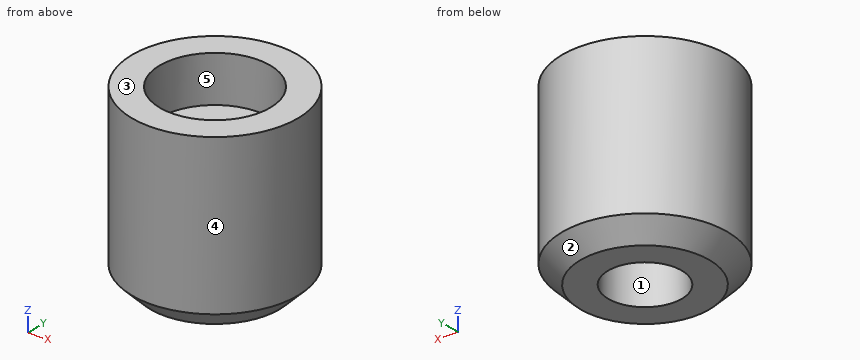
Autodesk Inventor part; units mm, degrees
ref_plane "YZ Plane" through (0, 0, 0) normal (1, 0, 0) x (0, 1, 0)
ref_plane "XZ Plane" through (0, 0, 0) normal (0, 1, 0) x (-1, 0, 0)
ref_plane "XY Plane" through (0, 0, 0) normal (0, 0, 1) x (1, 0, 0)
sketch "Skizze1" plane through (0, 0, 0) normal (0, 0, 1) x (1, 0, 0)
  circle A0 centre (0, 0) radius 2
  circle A1 centre (0, 0) radius 4.5
  dimension "d0" = 9
  dimension "d1" = 4
extrude "Extrusion1" add sketch "Skizze1" along normal blind 9.5
sketch "Skizze2" plane through (0, 0, 9.5) normal (0, 0, 1) x (1, 0, 0)
  circle A0 centre (0, 0) radius 3
  dimension "d4" = 6
extrude "Extrusion2" cut sketch "Skizze2" against normal blind 2.5
chamfer "Fase1" distance 1 angle 45 1 edges at (-4.5, 0, 0)
sketch "Skizze3" plane through (0, 0, 7) normal (0, 0, 1) x (1, 0, 0)
  circle A0 centre (0, 0) radius 2
  circle A1 centre (0, 0) radius 3
extrude "Extrusion3" add sketch "Skizze3" against normal blind 0.4 contours A0
properties part number "Mag4mmWelle" material "ABS-Kunststoff"
Verification items for the finished model (mm, model axes). Face numbers are marked on the shaded views. A direction names the side the tool comes from. Coordinates: 2 decimals unless noted, no trailing zeros. Order: outer loops, then holes, each group sorted by start corner. A loop starts at its lowest first (then second) coordinate and runs counter-clockwise, first axis right, second up. Notation, with made-up numbers: M 65.25,35 L 73.25,35 A35 cw 73.25,71 Z; hole C 75,-2 d7. An arc over 180 degrees is marked long. One line per item, written item: value. Start each with the question number.
Item 1: Sectioned sample at C-C on z = 8.5. Record the cut outline in (x, y), then the cut area to 3 significant figures.
Item 2: Access from +Z, -Z, +X, -X, +Y, -Y to the whole of each face (thin tool, end or side, straight path). Record for the marked faces 4 and 5.
Item 3: Sectioned sample at A-A on x = 0. Record the cut outline in (y, z).
Item 4: Mould release check, pull along Y, two halves, no side actions. Record for the marked faces 1, 2 and 3: pulls with the +Y half, pulls with the -Y half, needs draft (parallel to the pull), parting line crosses it, or undercut.
Item 5: Sectioned sample at B-B on z = 5.25. Record the cut outline in (x, y), then the cut area to 3 significant figures.
Item 6: Depth check by flat-ended pin: P1, Ø1, axis at x = -2, z = 5.5, coming from the -Y side; P2, Ø3.5, axis at x = 0, y = 0, coming from the +Z side; P3, Ø1.2, axis at x = 0.5, y = -0.5, coming from the -Z side. Enter the tip coordinate at first touch or a pass-through.
Item 7: Thickness scan on probe 1 along Y at (x, z) = (0, 7.85); probe 2 along Z at (x, y) = (-1.75, -0.75); probe 3 along Y at (x, z) = (0, 3.75). Record the ranges inside material, lowest first.
Calculated:
1. outline: C 0,0 d9; hole C 0,0 d6
1. area: 35.3 mm^2
2. face 4: +Z, -Z
2. face 5: +Z
3. outline: M -4.5,1 L -3.5,0 L -2,0 L -2,6.6 L 2,6.6 L 2,0 L 3.5,0 L 4.5,1 L 4.5,9.5 L 3,9.5 L 3,7 L -3,7 L -3,9.5 L -4.5,9.5 Z
4. face 1: undercut
4. face 2: parting line crosses it
4. face 3: needs draft
5. outline: C 0,0 d9; hole C 0,0 d4
5. area: 51.1 mm^2
6. P1: y = -4.24
6. P2: z = 7
6. P3: z = 6.6
7. probe 1: -4.5 to -3, 3 to 4.5
7. probe 2: 6.6 to 7
7. probe 3: -4.5 to -2, 2 to 4.5
